Can you work these out from the model? Positions are in its coordinate system, mm. A direction names the side the tool comes from. Give positions to 0.01 mm unless a question says otherwise; leave off trailing zeros. Loops run counter-clockwise (first coordinate to the right, second up) from the corner with the lowest first, then second, coordinate; pieces in that order, holes last. Notation, with made-up numbers: (33.5, -11.5) -> (53.5, -11.5) arc R21 cw to (53.5, -4.5) -> close; hole circle Ø4 at (5, 38.25). An arc over 180 degrees is marked (long way). Return JSON: item names as keys, results as strings. Group by question number.
Q1. Which directions (+Z, -Z, +X, -X, +Y, -Y) give clear straight access to the entire face, cutting with the end or side of a thin tool? Please do faces 1 (the cylindrical face through (20.14, -3.173, 0.705)), 2 (the flat face through (5.07, 57.05, -23.63)).
Q2. Thinking about a two-plate mould opening in Z: for faces 3 (the flat face through (10, 2, -24)), 4 (the cylindrical face through (5.1, 22.7, 15.3)), which applies, pulls with the +Z half, pulls with the -Z half, needs draft (parallel to the pull), parting line crosses it, or undercut?
Q3. Suppose I cut it at B-B, the plane z = 60. Count the separate pieces of the cut face and the enclosed holes in it, and give its area (3 significant figures).
Q4. Suppose I cut it at A-A, the plane x = 15. Please give me the cut outline in (y, z), and give its area (3 significant figures).
Q5. Will these pins go through, and if not, where does the flat tip stop? pin 1 (5 mm diameter, centred on y = -69, z = -63, fed in from -X); pin 2 (3.5 mm diameter, centred on x = 20.16, z = 0, fed in from -Y); pin 3 (3 mm diameter, centred on y = 1, z = 1, fed in from +X); pin 4 (3 mm diameter, centred on x = 5, z = -76, fed in from -Y).
Q6. I need wall thicknesses on line 1 along X through (y, z) = (4, 0); line 2 along Y through (x, z) = (23, 0); line 3 along Y through (x, z) = (6, 56.5). Which ranges of each line are inside material? Lowest first, please. Write a range as [from, to].
```python
from build123d import *

# Parameters (mm, degrees)
SKETCH1_R           = 115.22
BOSS_EXTRUDE1_DEPTH = 10
FILLET1_R           = 0.5
CUT_EXTRUDE1_DEPTH  = 10
SKETCH3_R           = 7.5
BOSS_EXTRUDE2_DEPTH = 20
FILLET3_R           = 1
SKETCH4_R           = 3.25
CUT_EXTRUDE2_DEPTH  = 20
SKETCH5_R           = 1.6
CUT_EXTRUDE4_DEPTH  = 20


with BuildPart() as part:
    # Sketch1 → Boss-Extrude1 (new body)
    with BuildSketch(Plane(origin=(0, 0, 0), x_dir=(0, 0, -1), z_dir=(1, 0, 0))):
        Circle(SKETCH1_R)
    extrude(amount=BOSS_EXTRUDE1_DEPTH)

    # Fillet1
    fillet1_edges = [part.edges().sort_by_distance(p)[0] for p in [
        (0, 0, 115.22),
        (10, 0, 115.22),
    ]]
    fillet(fillet1_edges, radius=FILLET1_R)

    # Sketch2 → Cut-Extrude1 (cut)
    with BuildSketch(Plane(origin=(10, 0, 0), x_dir=(0, 0, -1), z_dir=(1, 0, 0))):
        with BuildLine():
            Line((-89.710835252, 37.159444653), (-25.292265207, 10.476399272))
            ThreePointArc((-25.292265207, 10.476399272), (-26.850125531, 5.340822034), (-27.376150588, 0))
            Line((-27.376150588, 0), (-97.102308359, 0))
            ThreePointArc((-97.102308359, 0), (-95.236514731, 18.943720606), (-89.710835252, 37.159444653))
        make_face()
        with BuildLine():
            Line((-68.661700709, 68.661700709), (-19.357861723, 19.357861723))
            ThreePointArc((-19.357861723, 19.357861723), (-15.209374361, 22.762437316), (-10.476399272, 25.292265207))
            Line((-10.476399272, 25.292265207), (-37.159444653, 89.710835252))
            ThreePointArc((-37.159444653, 89.710835252), (-53.947152082, 80.737618685), (-68.661700709, 68.661700709))
        make_face()
        with BuildLine():
            Line((0, 97.102308359), (0, 27.376150588))
            ThreePointArc((0, 27.376150588), (5.340822034, 26.850125531), (10.476399272, 25.292265207))
            Line((10.476399272, 25.292265207), (37.159444653, 89.710835252))
            ThreePointArc((37.159444653, 89.710835252), (18.943720606, 95.236514731), (0, 97.102308359))
        make_face()
        with BuildLine():
            Line((68.661700709, 68.661700709), (19.357861723, 19.357861723))
            ThreePointArc((19.357861723, 19.357861723), (22.762437316, 15.209374361), (25.292265207, 10.476399272))
            Line((25.292265207, 10.476399272), (89.710835252, 37.159444653))
            ThreePointArc((89.710835252, 37.159444653), (80.737618685, 53.947152082), (68.661700709, 68.661700709))
        make_face()
        with BuildLine():
            Line((97.102308359, 0), (27.376150588, 0))
            ThreePointArc((27.376150588, 0), (26.850125531, -5.340822034), (25.292265207, -10.476399272))
            Line((25.292265207, -10.476399272), (89.710835252, -37.159444653))
            ThreePointArc((89.710835252, -37.159444653), (95.236514731, -18.943720606), (97.102308359, 0))
        make_face()
        with BuildLine():
            Line((68.661700709, -68.661700709), (19.357861723, -19.357861723))
            ThreePointArc((19.357861723, -19.357861723), (15.209374361, -22.762437316), (10.476399272, -25.292265207))
            Line((10.476399272, -25.292265207), (37.159444653, -89.710835252))
            ThreePointArc((37.159444653, -89.710835252), (53.947152082, -80.737618685), (68.661700709, -68.661700709))
        make_face()
        with BuildLine():
            Line((0, -97.102308359), (0, -27.376150588))
            ThreePointArc((0, -27.376150588), (-5.340822034, -26.850125531), (-10.476399272, -25.292265207))
            Line((-10.476399272, -25.292265207), (-37.159444653, -89.710835252))
            ThreePointArc((-37.159444653, -89.710835252), (-18.943720606, -95.236514731), (0, -97.102308359))
        make_face()
        with BuildLine():
            Line((-68.661700709, -68.661700709), (-19.357861723, -19.357861723))
            ThreePointArc((-19.357861723, -19.357861723), (-22.762437316, -15.209374361), (-25.292265207, -10.476399272))
            Line((-25.292265207, -10.476399272), (-89.710835252, -37.159444653))
            ThreePointArc((-89.710835252, -37.159444653), (-80.737618685, -53.947152082), (-68.661700709, -68.661700709))
        make_face()
    extrude(amount=-CUT_EXTRUDE1_DEPTH, mode=Mode.SUBTRACT)

    # Sketch3 → Boss-Extrude2 (add)
    with BuildSketch(Plane(origin=(10, 0, 0), x_dir=(0, 0, -1), z_dir=(1, 0, 0))):
        Circle(SKETCH3_R)
    extrude(amount=BOSS_EXTRUDE2_DEPTH)

    # Fillet3
    fillet3_edges = [part.edges().sort_by_distance(p)[0] for p in [
        (10, 0, 7.5),
    ]]
    fillet(fillet3_edges, radius=FILLET3_R)

    # Sketch4 → Cut-Extrude2 (cut)
    with BuildSketch(Plane(origin=(30, 0, 0), x_dir=(0, 0, -1), z_dir=(1, 0, 0))):
        Circle(SKETCH4_R)
    extrude(amount=-CUT_EXTRUDE2_DEPTH, mode=Mode.SUBTRACT)

    # Sketch5 → Cut-Extrude4 (cut)
    with BuildSketch(Plane(origin=(0, 0, 0), x_dir=(1, 0, 0), z_dir=(0, 1, 0))):
        with Locations(Location((20.158087078, 0, 0), (0, 0, 90))):
            Circle(SKETCH5_R)
    extrude(amount=CUT_EXTRUDE4_DEPTH, mode=Mode.SUBTRACT)


solid = part.part
```
Ans:
{
 "1": {"face 1": "+X", "face 2": "+X, -X"},
 "2": {"face 3": "needs draft", "face 4": "undercut"},
 "3": {"separate pieces": "4", "enclosed holes": "0", "area": "1,200 mm^2"},
 "4": {"outline": "circle Ø15 at (0, 0); hole circle Ø6.5 at (0, 0)", "area": "144 mm^2"},
 "5": {"pin 1": "passes through", "pin 2": "stops at y = -7.5", "pin 3": "stops at x = 10", "pin 4": "stops at y = -87.89"},
 "6": {"line 1": "x = [0, 18.56], [21.76, 30]", "line 2": "y = [-7.5, -3.25], [3.25, 7.5]", "line 3": "y = [-100.42, -56.5], [-23.4, 0], [23.4, 56.5], [78.97, 100.42]"}
}
